from build123d import *

# Parameters (mm, degrees)
SKETCH1_R           = 3.81
BOSS_EXTRUDE1_DEPTH = 5.08
SKETCH2_R           = 2.54
BOSS_EXTRUDE2_DEPTH = 32.512
FILLET1_R           = 0.508


with BuildPart() as part:
    # Sketch1 → Boss-Extrude1 (new body)
    with BuildSketch(Plane.XY):
        Circle(SKETCH1_R)
        Polygon((1.905, 1.099852263), (0, 2.199704526), (-1.905, 1.099852263), (-1.905, -1.099852263), (0, -2.199704526), (1.905, -1.099852263), align=None, mode=Mode.SUBTRACT)
    extrude(amount=BOSS_EXTRUDE1_DEPTH)

    # Sketch2 → Boss-Extrude2 (add)
    with BuildSketch(Plane.XY.offset(5.08)):
        Circle(SKETCH2_R)
    extrude(amount=BOSS_EXTRUDE2_DEPTH)

    # Fillet1
    fillet1_edges = [part.edges().sort_by_distance(p)[0] for p in [
        (-2.54, 0, 37.592),
    ]]
    fillet(fillet1_edges, radius=FILLET1_R)


solid = part.part
Verification items for the finished model (mm, model axes). A direction names the side the tool comes from. Round coordinates to 2 decimals unless told otherwise and drop trailing zeros. Loops run counter-clockwise (first coordinate to the right, second up) from the corner with the lowest first, then second, coordinate; pieces in that order, holes last. Notation, with made-up numbers: M 61.5,87.5 L 116.5,87.5 A16 ccw 116.5,117.5 Z; hole C -27,42.5 d11. An arc over 180 degrees is marked long. Write each question's results on one line, items separated by ' | '.
1) Section check A-A on z = 2.5. Record the boundary of the cut face in (x, y) (3 decimals), then the cut area to 3 significant figures.
Checks:
outline: C 0,0 d7.62; hole M -1.905,-1.1 L 0,-2.2 L 1.905,-1.1 L 1.905,1.1 L 0,2.2 L -1.905,1.1 Z | area: 33.0 mm2
2) Section check D-D on x = 3.25. Record the boundary of the cut face in (y, z).
Checks:
outline: M -1.99,0 L 1.99,0 L 1.99,5.08 L -1.99,5.08 Z
3) Section check B-B on y = 0. Record the boundary of the cut face in (x, z) (3 decimals).
Checks:
outline: M -3.81,0 L -1.905,0 L -1.905,5.08 L 1.905,5.08 L 1.905,0 L 3.81,0 L 3.81,5.08 L 2.54,5.08 L 2.54,37.084 A0.508 ccw 2.032,37.592 L -2.032,37.592 A0.508 ccw -2.54,37.084 L -2.54,5.08 L -3.81,5.08 Z
4) Access from +Z, -Z, +X, -X, +Y, -Y to the whole of each face (thin tool, end or side, straight path). Record for faces 4 (the flat face through (0, 0, 37.592)), 5 (the flat face through (0, 3, 5.08)), 6 (the flat face through (-0.939, 1.657, 2.504)).
Checks:
face 4: +Z, +X, -X, +Y, -Y | face 5: +Z | face 6: -Z
5) Scan lines: L1, parallel to Z at x = 1, y = 3; L2, parallel to Z at x = 1, y = 1; L3, parallel to Y at x = 0, z = 24.5. Record each from-to range of solid material in increasing order. Write a range as from..to.
Checks:
L1: z = 0..5.08 | L2: z = 5.08..37.59 | L3: y = -2.54..2.54
6) Mould release check, pull along Y, two halves, no side actions. Record for faces 1 (the flat face through (0.97, 1.64, 2.5)), 2 (the cylindrical face through (-0.83, -3.72, 2.5)), 3 (the flat face through (1, 2, 0)): released by +Y, released by -Y, zero draft, split by the parting line, or undercut.
Checks:
face 1: undercut | face 2: split by the parting line | face 3: zero draft
7) Section check C-C on z = 23. Record the boundary of the cut face in (x, y), then the cut area to 3 significant figures.
Checks:
outline: C 0,0 d5.08 | area: 20.3 mm2
8) Gauge pin test, flat ends, axial feed: P1, Ø1.5, axis at x = 3, y = 1.5, coming from the +Z side; P2, Ø1.1, axis at x = -0.5, y = 0.5, coming from the -Z side. Record the tip position at first contact, or that the pin passes through.
Checks:
P1: stops at z = 5.08 | P2: stops at z = 5.08
